Geometry check sheet. Reference: the model listing, model coordinates, mm. Face numbers are marked on the shaded views. A direction names the side the tool comes from. Give positions to 0.01 mm unless a question says otherwise; leave off trailing zeros. Order: outer loops, then holes, each group sorted by start corner. A loop starts at its lowest first (then second) coordinate and runs counter-clockwise, first axis right, second up. Notation, with made-up numbers: M -17.5,10.25 L 41.5,10.25 A6 ccw 41.5,15.25 Z; hole C 32.25,-16 d11. An arc over 180 degrees is marked long. Put each result on its own line as item: value. Start each with the question number.
Q1. Go/stop test with flat-tipped pins: pin 1 (4 mm diameter, centred on x = 32, z = 22, fed in from +Y); pin 2 (5 mm diameter, centred on x = 18, y = -14, fed in from -Z); pin 3 (4 mm diameter, centred on y = -6.5, z = 14.5, fed in from +X); pin 4 (1 mm diameter, centred on y = -10.5, z = 13.5, fed in from +X). Record where each tip stops, or that it passes through.
Q2. Section check B-B on x = 15.5. Record the cut outline in (y, z).
Q3. Material ranges on L1, parallel to Y at x = 15.5, z = 4; L2, parallel to X at y = 18.6, z = 20; L3, parallel to Y at x = 0, z = 1.9, recorded low to high.
Q4. Mould release check, pull along Y, two halves, no side actions. Record for the marked faces 1, 2 and 3: +Y half, -Y half, draft (parallel to the pull), parting line (faces both ways), or undercut.
Q5. Section check A-A on x = -32. Record the cut outline in (y, z), then the cut area to 3 significant figures.
Q6. Section check D-D on y = 0. Record the cut outline in (x, z), then the cut area to 3 significant figures.
Q7. Section check C-C on y = -15.5. Record the cut outline in (x, z), then the cut area to 3 significant figures.
Q8. Access from +Z, -Z, +X, -X, +Y, -Y to the whole of each face (thin tool, end or side, straight path). Record for the marked faces 4, 5, 6 and 7.
Autodesk Fusion 360 part; units mm, degrees
sketch "スケッチ1" plane through (0, 0, 0) normal (0, 0, 1) x (1, 0, 0)
  line L0 (-26.5, 47) -> (26.5, 47)
  line L1 (26.5, 47) -> (26.5, -21)
  line L2 (26.5, -21) -> (-26.5, -21)
  line L3 (-26.5, -21) -> (-26.5, 47)
  circle A0 centre (0, 0) radius 11.2
  circle A1 centre (-15.5, -15.5) radius 1.75
  circle A2 centre (15.5, -15.5) radius 1.75
  circle A3 centre (15.5, 15.5) radius 1.75
  circle A4 centre (-15.5, 15.5) radius 1.75
  line L4 (21.5, 17) -> (37.5, 17)
  line L5 (37.5, 17) -> (37.5, 22)
  line L6 (37.5, 22) -> (21.5, 22)
  line L7 (21.5, 22) -> (21.5, 17)
  circle A5 centre (20, 37) radius 2.7
  line L8 (0, 0) -> (0, 47) construction
  line L9 (-37.5, 22) -> (-21.5, 22)
  line L10 (-21.5, 22) -> (-21.5, 17)
  line L11 (-21.5, 17) -> (-37.5, 17)
  line L12 (-37.5, 17) -> (-37.5, 22)
  circle A6 centre (-20, 37) radius 2.7
  line L13 (26.5, 39.7) -> (20, 39.7)
  line L14 (26.5, 34.3) -> (20, 34.3)
  line L15 (-26.5, 34.3) -> (-20, 34.3)
  line L16 (-26.5, 39.7) -> (-20, 39.7)
  dimension "d1" = 53
  dimension "d2" = 68
  dimension "d3" = 26.5
  dimension "d4" = 21
  dimension "d5" = 22.4
  dimension "d6" = 3.5
  dimension "d7" = 15.5
  dimension "d8" = 15.5
  dimension "d10" = 360
  dimension "d11" = 16
  dimension "d12" = 5
  dimension "d13" = 11
  dimension "d14" = 25
  dimension "d15" = 5.4
  dimension "d16" = 10
  dimension "d17" = 6.5
extrude "押し出し1" add sketch "スケッチ1" along normal blind 5 contours L0 L1 L2 L3 L4 L6 L7 A5 L9 L10 L11 A6 L13 L14 L15 L16
extrude "押し出し2" add sketch "スケッチ1" along normal blind 30 contours L3 L9 L10 L11 | L3 L9 L11 L12 | L1 L4 L5 L6 | L1 L4 L6 L7
chamfer "面取り1" distance 38 distance2 25 2 edges at (24, 17, 5) (-24, 17, 5) measured on face at (0.279, 27.7319, 5) measured on face at (0.279, 27.7319, 5)
fillet "フィレット1" radius 1 14 edges at (-37.5, 17, 15) (-37.5, 22, 15) (-26.5, -21, 2.5) (-26.5, 34.3, 2.5) (-26.5, 39.7, 2.5) (-26.5, 47, 2.5) (26.5, 47, 2.5) (26.5, 39.7, 2.5) (26.5, 34.3, 2.5) (37.5, 22, 15) (37.5, 17, 15) (21.5, 22, 17.5) (-21.5, 22, 17.5) (26.5, -21, 2.5)
hole "穴1" at (-32, 17, 20) direction (0, 1, 0) diameter 5.4 depth 11 tip angle 118
mirror "ミラー1" about plane through (0, 0, 0) normal (1, 0, 0) of "穴1"
equation "d3 = d1 / 2"
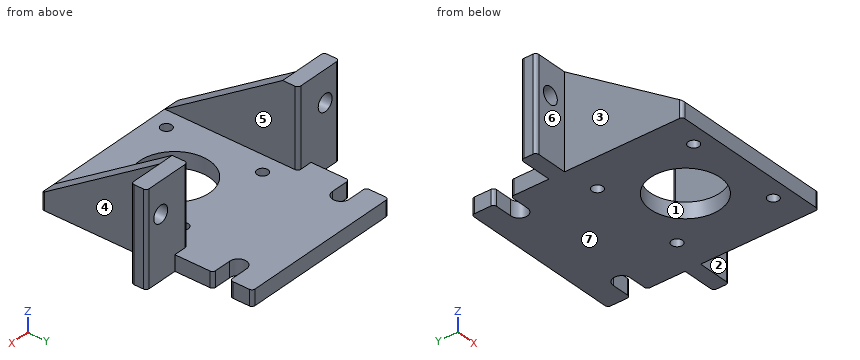
Results found:
1. pin 1: stops at y = 22
1. pin 2: stops at z = 0
1. pin 3: stops at x = 26.5
1. pin 4: passes through
2. outline: M -21,0 L -17.25,0 L -17.25,5 L -21,5 Z; M -13.75,0 L 13.75,0 L 13.75,5 L -13.75,5 Z; M 17.25,0 L 47,0 L 47,5 L 17.25,5 Z
3. L1: y = -21 to -17.25, -13.75 to 13.75, 17.25 to 47
3. L2: x = -37.5 to -34.7, -29.3 to -21.5, 21.5 to 29.3, 34.7 to 37.5
3. L3: y = -21 to -11.2, 11.2 to 47
4. face 1: undercut
4. face 2: -Y half
4. face 3: draft
5. outline: M 17,0 L 22,0 L 22,17.3 L 17,17.3 Z; M 17,22.7 L 22,22.7 L 22,30 L 17,30 Z
5. area: 123 mm^2
6. outline: M -26.5,0 L -11.2,0 L -11.2,5 L -21.5,5 L -21.5,18.81 L -26.5,18.81 Z; M 11.2,0 L 26.5,0 L 26.5,18.81 L 21.5,18.81 L 21.5,5 L 11.2,5 Z
6. area: 291 mm^2
7. outline: M -26.5,0 L -17.25,0 L -17.25,5 L -21.5,5 L -21.5,8.61 L -26.5,8.61 Z; M -13.75,0 L 13.75,0 L 13.75,5 L -13.75,5 Z; M 17.25,0 L 26.5,0 L 26.5,8.61 L 21.5,8.61 L 21.5,5 L 17.25,5 Z
7. area: 266 mm^2
8. face 4: +Z, -Z, +X, -Y
8. face 5: +Z, +Y, -Y
8. face 6: +Z, -Z, -X, -Y
8. face 7: -Z, +X, -X, +Y, -Y
